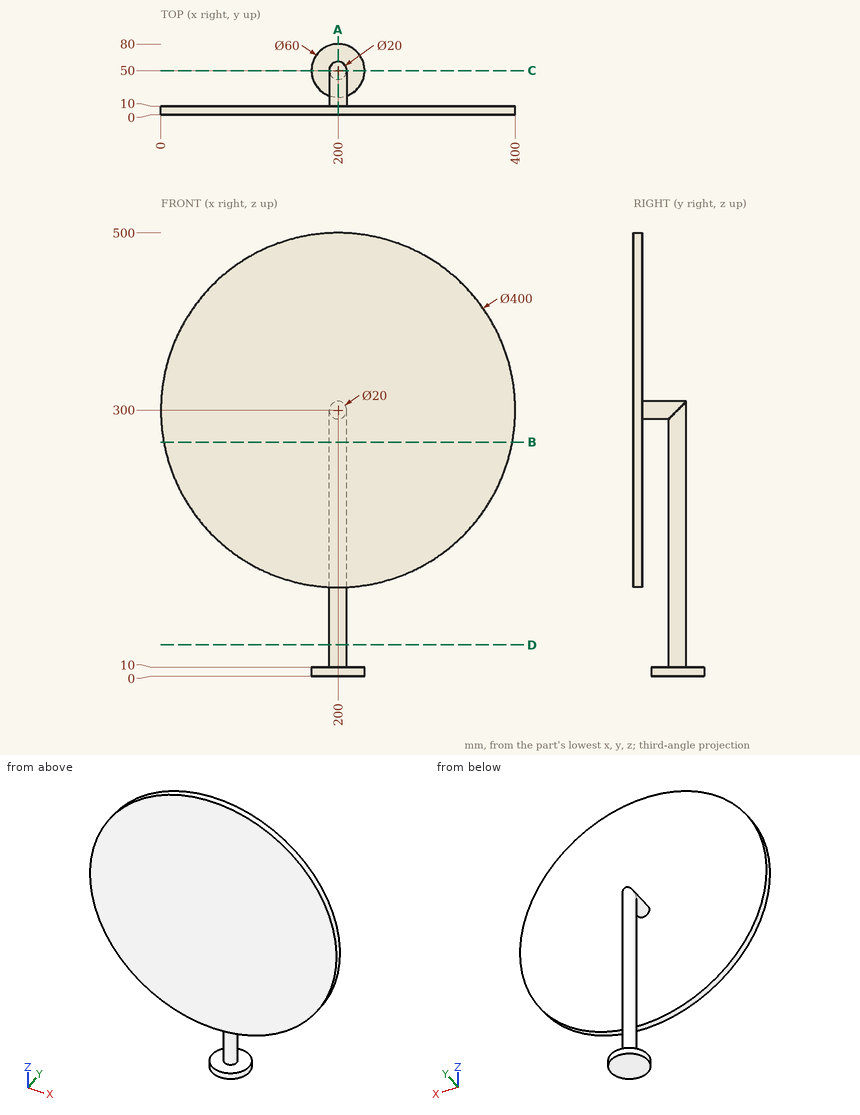
The drawing under review shows one solid part. Ordinate dimensions are in mm from its lowest x, y, z. Round coordinates to 2 decimals unless told otherwise and drop trailing zeros. Order: outer loops, then holes, each group sorted by start corner. A loop starts at its lowest first (then second) coordinate and runs counter-clockwise, first axis right, second up. Notation, with made-up numbers: M 58,59 L 62,59 A24 ccw 62,93 Z; hole C 19.5,36.5 d8. An arc over 180 degrees is marked long. Answer as CSV lines item,"result". Start each with the question number.
1) Add section D-D (z = 35). Give the boundary of the cut face in (x, y).
2) Add section B-B (z = 264). Give the boundary of the cut face in (x, y).
3) Add section A-A (x = 200). Give the boundary of the cut face in (y, z).
4) Add section C-C (y = 50). Give the boundary of the cut face in (x, z).
5) For pin 1 Ø12 at (x, z) = (299, 331.5) entering from +Y; pin 2 Ø18 at (x, y) = (208, 45.5) entering from +Z, all flat-tipped, find the tip position at first contact; note any pin that passes through.
6) Wall thickness on line 1 along Y through (x, z) = (124, 276); line 2 along X through (y, z) = (5, 453): over which ranges is each line inside the solid? List them lowest first. Write a range as [from, to].
Resolved:
1,outline,"C 200,50 d20"
2,outline,"M 3.27,0 L 396.73,0 L 396.73,10 L 3.27,10 Z; C 200,50 d20"
3,outline,"M 0,100 L 10,100 L 10,290 L 40,290 L 40,10 L 20,10 L 20,0 L 80,0 L 80,10 L 60,10 L 60,310 L 10,310 L 10,500 L 0,500 Z"
4,outline,"M 170,0 L 230,0 L 230,10 L 210,10 L 210,300 A10 ccw 190,300 L 190,10 L 170,10 Z"
5,pin 1,"y = 10"
5,pin 2,"z = 310"
6,line 1,"[0, 10]"
6,line 2,"[71.19, 328.81]"
